Study the drawing (mm; zero at the part's minimum x, y, z) and answer. Coordinates: 2 decimals unless noted, no trailing zeros. Order: outer loops, then holes, each group sorted by start corner. A loop starts at its lowest first (then second) coordinate and runs counter-clockwise, first axis right, second up. Notation, with made-up numbers: M 2,75 L 21,75 A30 ccw 21,110 Z; hole C -23.5,-33 d10. An arc over 180 degrees is marked long. One line per item, written item: value. Start each with the question number.
Q1. Straight lines are drawn through the part: line 1 along X through (y, z) = (99, 100); line 2 along X through (y, z) = (154.5, 69). For each, find the intervals that lie inside material, in ascending order. Write a range as [from, to].
Q2. The part is cut by section A-A on z = 100. Give the vertices of the cut face in (x, y).
Q3. The part is cut by section B-B on x = 100. Give the vertices of the cut face in (y, z).
Q4. The part is cut by section C-C on y = 32.5. Give the vertices of the cut face in (x, z).
Q5. Each of these flat-tipped pins is pushed along its axis until it touches: pin 1 Ø4 at (y, z) = (27, 82.5) entering from -X; pin 2 Ø5 at (y, z) = (107, 161) entering from -X; pin 3 Ø6 at (x, y) = (78, 59.5) entering from -Z. Where does it stop, or does it pass through?
Q6. Determine the mould class of the marked faces 1 and 2 for opening direction X: pulls with the +X half, pulls with the -X half, needs draft (parallel to the pull), parting line crosses it, or undercut.
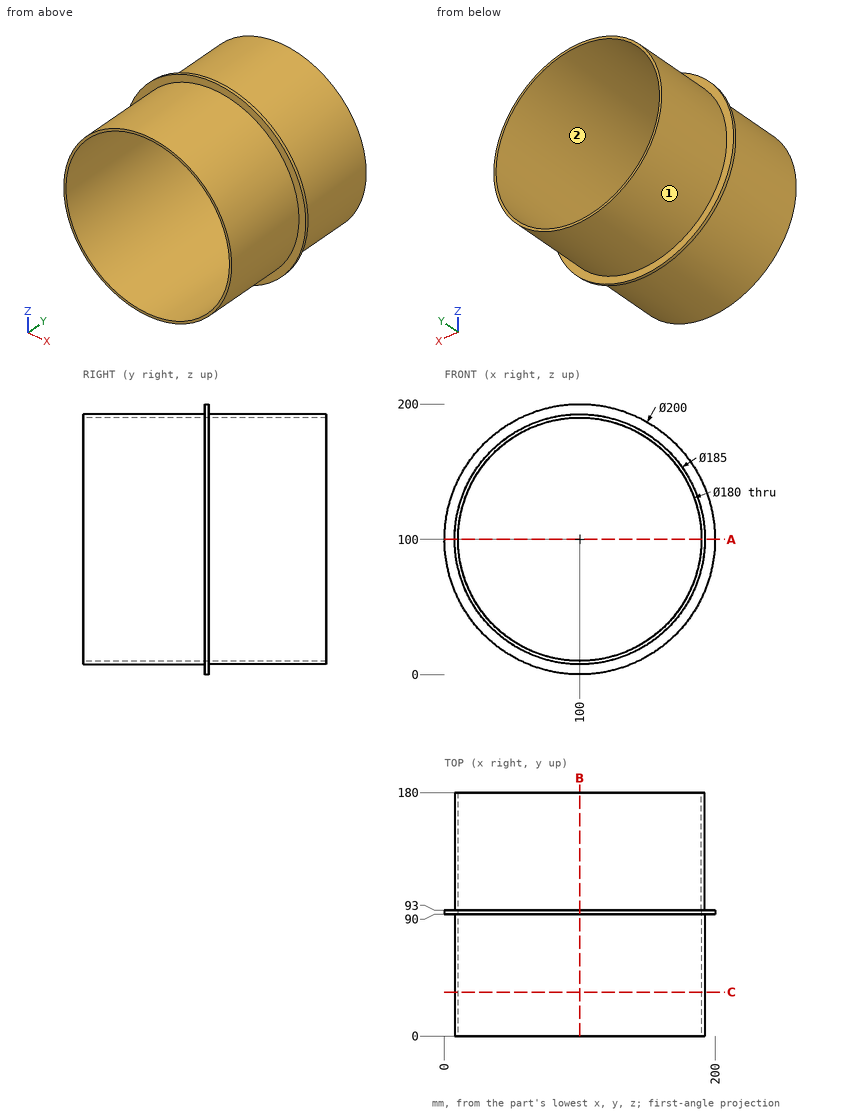
Output:
1. line 1: x = [7.5, 10], [190, 192.5]
1. line 2: x = [12.85, 15.51], [184.49, 187.15]
2. outline: M 0,90 L 7.5,90 L 7.5,0 L 10,0 L 10,180 L 7.5,180 L 7.5,93 L 0,93 Z; M 190,0 L 192.5,0 L 192.5,90 L 200,90 L 200,93 L 192.5,93 L 192.5,180 L 190,180 Z
3. outline: M 0,7.5 L 90,7.5 L 90,0 L 93,0 L 93,7.5 L 180,7.5 L 180,10 L 0,10 Z; M 0,190 L 180,190 L 180,192.5 L 93,192.5 L 93,200 L 90,200 L 90,192.5 L 0,192.5 Z
4. outline: C 100,100 d185; hole C 100,100 d180
5. pin 1: stops at x = 8.81
5. pin 2: stops at x = 28.35
5. pin 3: stops at z = 9.47
6. face 1: parting line crosses it
6. face 2: undercut
